```python
from build123d import *

# Parameters (mm, degrees)
ZAOKR_GLENIE1_R            = 0.6
SFAZOWANIE1_SIZE           = 0.6
WYTNIJ_WYCI_GNI_CIE1_DEPTH = 5


with BuildPart() as part:
    # ruba parametryczna → Obrót1 (revolve)
    with BuildSketch(Plane.XY):
        Polygon((0, 0), (0, 6.5), (-5.5, 6.5), (-5.5, 4), (-30.5, 4), (-30.5, 3), (-41.5, 3), (-41.5, 0), align=None)
    revolve(axis=Axis((0, 0, 0), (1, 0, 0)))

    # Zaokrąglenie1
    zaokr_glenie1_edges = [part.edges().sort_by_distance(p)[0] for p in [
        (0, -6.5, 0),
    ]]
    fillet(zaokr_glenie1_edges, radius=ZAOKR_GLENIE1_R)

    # Sfazowanie1
    sfazowanie1_edges = [part.edges().sort_by_distance(p)[0] for p in [
        (-41.5, -3, 0),
    ]]
    chamfer(sfazowanie1_edges, length=SFAZOWANIE1_SIZE)

    # Szkic2 → Wytnij-wyciągnięcie1 (cut)
    with BuildSketch(Plane(origin=(0, 0, 0), x_dir=(0, 0, -1), z_dir=(1, 0, 0))):
        Polygon((-2, -1.154700538), (0, -2.309401077), (2, -1.154700538), (2, 1.154700538), (0, 2.309401077), (-2, 1.154700538), align=None)
    extrude(amount=-WYTNIJ_WYCI_GNI_CIE1_DEPTH, mode=Mode.SUBTRACT)

    # Szkic3 → Wycięcie-obrót1 (revolve, cut)
    with BuildSketch(Plane(origin=(0, 0, 0), x_dir=(1, 0, 0), z_dir=(0, 1, 0))):
        with BuildLine():
            Line((-32, -3), (-30.5, -3))
            ThreePointArc((-30.5, -3), (-31.25, -2.661437828), (-32, -3))
        make_face()
    revolve(axis=Axis((3.805158027, 0, 0), (-1, 0, 0)), mode=Mode.SUBTRACT)


solid = part.part
```
The model under review builds one solid part; all positions refer to its coordinate system, in mm. A direction names the side the tool comes from. Coordinates: 2 decimals unless noted, no trailing zeros. Loops run counter-clockwise (first coordinate to the right, second up) from the corner with the lowest first, then second, coordinate; pieces in that order, holes last. Notation, with made-up numbers: (-39.75, 18.25) -> (0.25, 18.25) arc R17 ccw to (0.25, 32.25) -> close; hole circle Ø3 at (13.25, -1.75). An arc over 180 degrees is marked (long way). Answer as CSV lines item,"result".
Item 1: Take a section at C-C, the plane x = -36. State the section outline as (y, z) points, and give its area (3 significant figures).
Results below:
outline,"circle Ø6 at (0, 0)"
area,"28.3 mm2"
Item 2: Machinability: for faces 1 (the cylindrical face through (-18.175, -0.867, -3.905)), 2 (the flat face through (-2.46, 1.74, 0.99)), 3 (the flat face through (-41.5, 0, 0)), which of the approach directions +Z, -Z, +X, -X, +Y, -Y give a long, thin tool a straight path to every point of the face, cutting with its end or side? Answer none if there is none.
Results below:
face 1,"-X"
face 2,"+X"
face 3,"+Z, -Z, -X, +Y, -Y"
Item 3: Draft analysis for pull direction Y (two halves, no side actions). For faces 4 (the flat face through (-5.5, 3, 3)), 5 (the cylindrical face through (-3.084, -5.158, -3.955)), 6 (the flat face through (-2, 0, -2)), state which applies: +Y half, -Y half, draft (parallel to the pull), parting line (faces both ways), or undercut.
Results below:
face 4,"draft"
face 5,"parting line"
face 6,"undercut"
Item 4: Take a section at D-D, the plane x = -16. State the section outline as (y, z) points.
Results below:
outline,"circle Ø8 at (0, 0)"
Item 5: Take a section at A-A, the plane y = 0. State the section outline as (x, z) points.
Results below:
outline,"(-41.5, -2.4) -> (-40.9, -3) -> (-32, -3) arc R1 cw to (-30.5, -3) -> (-30.5, -4) -> (-5.5, -4) -> (-5.5, -6.5) -> (-0.6, -6.5) arc R0.6 ccw to (0, -5.9) -> (0, -2) -> (-5, -2) -> (-5, 2) -> (0, 2) -> (0, 5.9) arc R0.6 ccw to (-0.6, 6.5) -> (-5.5, 6.5) -> (-5.5, 4) -> (-30.5, 4) -> (-30.5, 3) arc R1 cw to (-32, 3) -> (-40.9, 3) -> (-41.5, 2.4) -> close"
Item 6: Take a section at B-B, the plane x = -3.5. State the section outline as (y, z) points, and give its area (3 significant figures).
Results below:
outline,"circle Ø13 at (0, 0); hole (-2.31, 0) -> (-1.15, -2) -> (1.15, -2) -> (2.31, 0) -> (1.15, 2) -> (-1.15, 2) -> close"
area,"119 mm2"
Item 7: Insertion check: pin 1 (2 mm diameter, centred on y = 0.5, z = 0.5, fed in from +X); pin 2 (2 mm diameter, centred on y = -5, z = -3.5, fed in from -X); pin 3 (1 mm diameter, centred on x = -5.5, z = 4, fed in from -Y). Each pin has a flat end and moves straight along its axis. Give the tip position at first contact, or say it passes through.
Results below:
pin 1,"stops at x = -5"
pin 2,"stops at x = -5.5"
pin 3,"stops at y = -5.48"
Item 8: For L1, parallel to X at y = 5.25, z = 0.75; L2, parallel to Z at x = -6.5, y = -2.25; L3, parallel to Z at x = -23, y = 0.25, list the stretches that pass through material, from the lowest coordinate up.
Results below:
L1,"x = -5.5 to 0"
L2,"z = -3.31 to 3.31"
L3,"z = -3.99 to 3.99"
